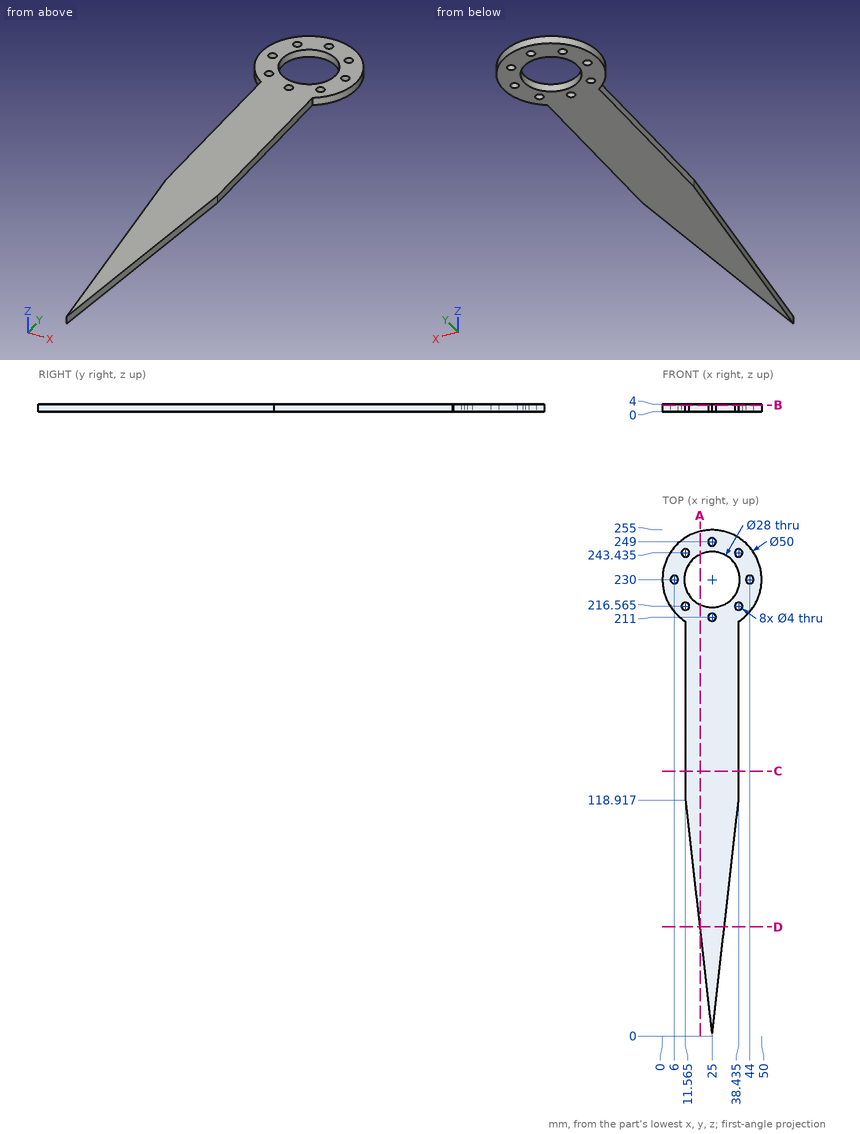
Geometry check sheet. Reference: drawing and pictorial views, mm from the part's lowest x, y, z. Coordinates: 2 decimals unless noted, no trailing zeros. Order: outer loops, then holes, each group sorted by start corner. A loop starts at its lowest first (then second) coordinate and runs counter-clockwise, first axis right, second up. Notation, with made-up numbers: (50, 9.25) - (59, 9.25) arc R27 ccw to (59, 25.25) - close; hole circle Ø6 at (3.25, -14.75). An arc over 180 degrees is marked (long way). One line per item, written item: value.
(1) Sectioned sample at A-A (x = 19). Enter the section's corners in (y, z).
Data:
outline: (53.11, 0) - (217.35, 0) - (217.35, 4) - (53.11, 4) - close; (242.65, 0) - (254.27, 0) - (254.27, 4) - (242.65, 4) - close
(2) Thickness scan on probe 1 along X at (y, z) = (128, 1.8) (3 decimals); probe 2 along X at (y, z) = (101, 3.45); probe 3 along Y at (x, z) = (9.5, 1.15) (1 decimal). Record the ranges inside material, lowest first. Write a range as from..to.
Data:
probe 1: x = 11.565..38.435
probe 2: x = 13.59..36.41
probe 3: y = 210.4..249.6
(3) Sectioned sample at B-B (z = 3.4). Count the separate pieces of the cut face and the enclosed holes in it, and give its area (3 significant figures).
Data:
separate pieces: 1
enclosed holes: 9
area: 5,190 mm^2
(4) Sectioned sample at D-D (y = 55). Enter the section's corners in (x, z), and give its area (3 significant figures).
Data:
outline: (18.79, 0) - (31.21, 0) - (31.21, 4) - (18.79, 4) - close
area: 49.7 mm^2
(5) Sectioned sample at C-C (y = 133.5). Enter the section's corners in (x, z) (3 decimals), and give its area (4 significant figures).
Data:
outline: (11.565, 0) - (38.435, 0) - (38.435, 4) - (11.565, 4) - close
area: 107.5 mm^2
(6) Depth check by flat-ended pin: pin 1 Ø4.5 at (x, y) = (11.56, 216.56) entering from +Z; pin 2 Ø3 at (x, y) = (38.44, 243.44) entering from +Z; pin 3 Ø1.2 at (y, z) = (160, 2) entering from +X (3 decimals); pin 4 Ø2 at (x, z) = (36, 1.5) entering from +Y. Enter the tip coordinate at first touch or a pass-through.
Data:
pin 1: stops at z = 4
pin 2: passes through
pin 3: stops at x = 38.435
pin 4: stops at y = 252.91
